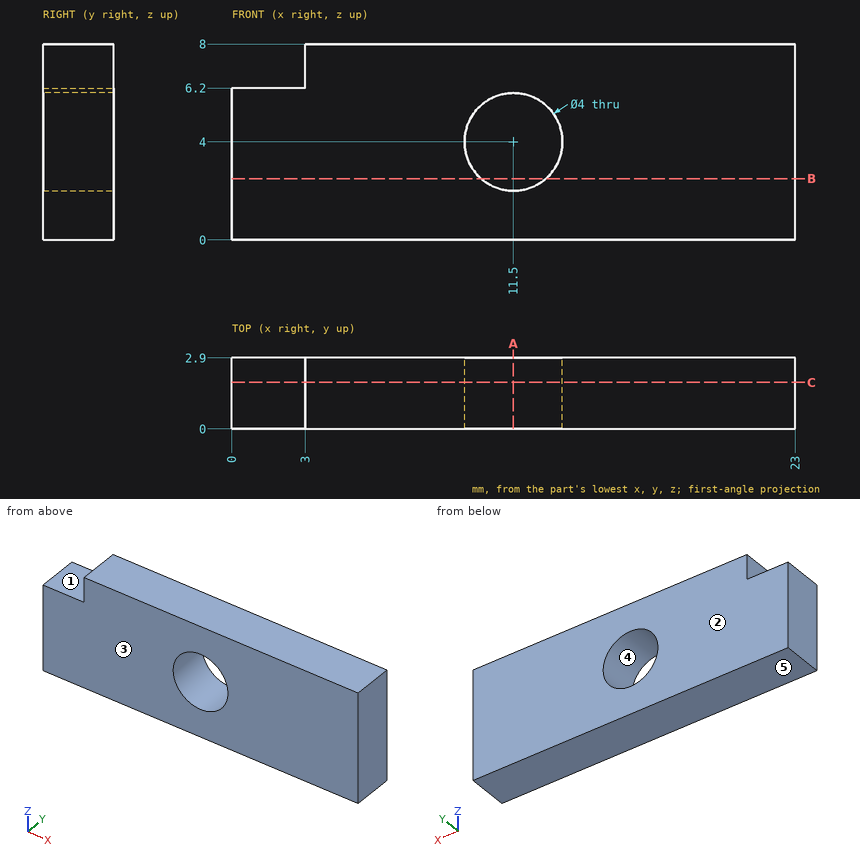
Geometry: see drawing. Coordinates: mm, zero at the bounding-box minimum. A direction names the side the tool comes from. Round coordinates to 2 decimals unless told otherwise and drop trailing zeros. Write each loop counter-clockwise with the first axis right and the second up, starting at its lowest first coordinate (ties: lowest second). Pieces come first, ordered by that corner, then holes. Notation, with made-up numbers: (0, 70) -> (7, 70) arc R29 ccw to (7, 98) -> close; hole circle Ø7 at (74, -19.75). An arc over 180 degrees is marked (long way). Answer as CSV lines item,"result".
1. Reachability of the marked faces 1 and 2 from +Z, -Z, +X, -X, +Y, -Y: full face, straight path, thin tool, end or side. Return the list, or none.
Geometry says:
face 1,"+Z, -X, +Y, -Y"
face 2,"+Z, -Z, +X, -X, +Y"
2. Contact query for flat-ended pins moving along their axis: P1, Ø1.4, axis at y = 1, z = 7.5, coming from the -X side; P2, Ø1.4, axis at x = 1.5, y = 2, coming from the +Z side. Output: stop coordinate, or through.
Geometry says:
P1,"stops at x = 3"
P2,"stops at z = 6.2"
3. Section B-B (z = 2.5). Return the cut outline in (x, y), plus the area to 3 significant figures.
Geometry says:
outline,"(0, 0) -> (10.18, 0) -> (10.18, 2.9) -> (0, 2.9) -> close; (12.82, 0) -> (23, 0) -> (23, 2.9) -> (12.82, 2.9) -> close"
area,"59.0 mm^2"
4. Mould query, pull axis Z, two halves, no side actions, for the marked faces 3, 4 and 5. Classes: +Z half, -Z half, draft (parallel to the pull), parting line (faces both ways), or undercut.
Geometry says:
face 3,"draft"
face 4,"undercut"
face 5,"-Z half"
5. Section C-C (y = 1.9). Return the cut outline in (x, z), plus the area to 3 significant figures.
Geometry says:
outline,"(0, 0) -> (23, 0) -> (23, 8) -> (3, 8) -> (3, 6.2) -> (0, 6.2) -> close; hole circle Ø4 at (11.5, 4)"
area,"166 mm^2"
6. Section A-A (x = 11.5). Return the cut outline in (y, z).
Geometry says:
outline,"(0, 0) -> (2.9, 0) -> (2.9, 2) -> (0, 2) -> close; (0, 6) -> (2.9, 6) -> (2.9, 8) -> (0, 8) -> close"
7. Ray query, L1, parallel to Z at x = 11.5, y = 1.3; L2, parallel to X at y = 1.85, z = 4; L3, parallel to X at y = 2.55, z = 6.25. Return the intervals inside material, ascending. Write a range as [from, to].
Geometry says:
L1,"z = [0, 2], [6, 8]"
L2,"x = [0, 9.5], [13.5, 23]"
L3,"x = [3, 23]"
